```python
from build123d import *

# Parameters (mm, degrees)
SKETCH1_W           = 31
SKETCH1_H           = 26
BOSS_EXTRUDE1_DEPTH = 1.2
SKETCH3_W           = 1.2
SKETCH3_H           = 26
BOSS_EXTRUDE2_DEPTH = 33
SKETCH4_R           = 3.5
CUT_EXTRUDE1_DEPTH  = 1.2
SKETCH2_R           = 5
SKETCH2_R_2         = 2
CUT_EXTRUDE2_DEPTH  = 1.2
FILLET1_R           = 1
FILLET2_R           = 3


with BuildPart() as part:
    # Sketch1 → Boss-Extrude1 (new body)
    with BuildSketch(Plane(origin=(0, 0, 0), x_dir=(1, 0, 0), z_dir=(0, 1, 0))):
        Rectangle(SKETCH1_W, SKETCH1_H)
    extrude(amount=BOSS_EXTRUDE1_DEPTH)

    # Sketch3 → Boss-Extrude2 (add)
    with BuildSketch(Plane.XZ):
        with Locations((14.9, 0)):
            Rectangle(SKETCH3_W, SKETCH3_H)
    extrude(amount=BOSS_EXTRUDE2_DEPTH)

    # Sketch4 → Cut-Extrude1 (cut)
    with BuildSketch(Plane(origin=(15.5, 0, 0), x_dir=(0, 0, -1), z_dir=(1, 0, 0))):
        with BuildLine():
            Line((13, -33), (13, -20))
            ThreePointArc((13, -20), (9.192388155, -29.192388155), (0, -33))
            Line((0, -33), (13, -33))
        make_face()
        with BuildLine():
            Line((-13, -33), (0, -33))
            ThreePointArc((0, -33), (-9.192388155, -29.192388155), (-13, -20))
            Line((-13, -20), (-13, -33))
        make_face()
        with Locations((0, -20)):
            Circle(SKETCH4_R)
    extrude(amount=-CUT_EXTRUDE1_DEPTH, mode=Mode.SUBTRACT)

    # Sketch2 → Cut-Extrude2 (cut)
    with BuildSketch(Plane(origin=(0, 1.2, 0), x_dir=(1, 0, 0), z_dir=(0, 1, 0))):
        with Locations(Location((0, 0, 0), (0, 0, 270))):
            Circle(SKETCH2_R)
        with Locations(Location((-7.5, 8, 0), (0, 0, 270))):
            Circle(SKETCH2_R_2)
        with Locations(Location((6.5, 8, 0), (0, 0, 270))):
            Circle(SKETCH2_R_2)
        with Locations(Location((6.5, -8, 0), (0, 0, 90))):
            Circle(SKETCH2_R_2)
        with Locations(Location((-7.5, -8, 0), (0, 0, 90))):
            Circle(SKETCH2_R_2)
    extrude(amount=-CUT_EXTRUDE2_DEPTH, mode=Mode.SUBTRACT)

    # Fillet1
    fillet1_edges = [part.edges().sort_by_distance(p)[0] for p in [
        (15.5, 1.2, 0),
        (14.3, 0, 0),
    ]]
    fillet(fillet1_edges, radius=FILLET1_R)

    # Fillet2
    fillet2_edges = [part.edges().sort_by_distance(p)[0] for p in [
        (-15.5, 0.6, -13),
        (-15.5, 0.6, 13),
    ]]
    fillet(fillet2_edges, radius=FILLET2_R)


solid = part.part
```
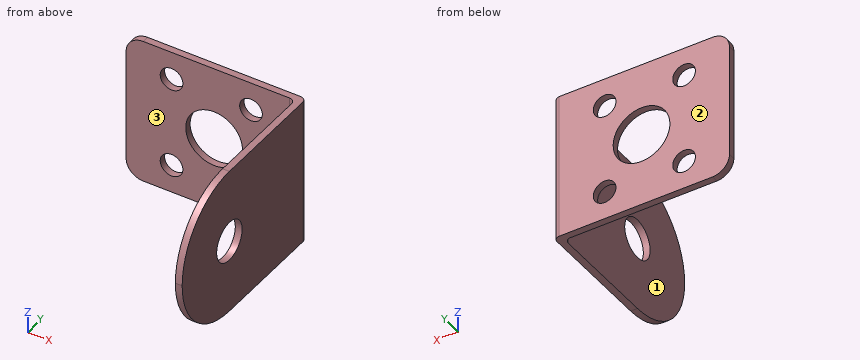
Can you work these out from the model? Positions are in its coordinate system, mm. Face numbers are marked on the shaded views. Coordinates: 2 decimals unless noted, no trailing zeros. Order: outer loops, then holes, each group sorted by start corner. A loop starts at its lowest first (then second) coordinate and runs counter-clockwise, first axis right, second up. Notation, with made-up numbers: (-29, -32.5) -> (-6, -32.5) arc R35 ccw to (-6, 2.5) -> close; hole circle Ø7 at (-39.75, 86). An arc over 180 degrees is marked (long way). Write each question's results on one line, items separated by ' | '.
Item 1: I want a section at A-A, the plane y = -18.5. Write out the boundary of the cut face in (x, z).
Results are:
outline: (14.3, -13) -> (15.5, -13) -> (15.5, -3.16) -> (14.3, -3.16) -> close; (14.3, 3.16) -> (15.5, 3.16) -> (15.5, 13) -> (14.3, 13) -> close
Item 2: If I drill on line 1 along X through (y, z) = (0.35, 8); line 2 along X through (y, z) = (0.8, 8); line 3 along Y through (x, z) = (-2.5, 8.25), over which ranges is the centre line in solid material (lowest first)?
Results are:
line 1: -15.5 to -9.5, -5.5 to 4.5, 8.5 to 15.49 | line 2: -15.5 to -9.5, -5.5 to 4.5, 8.5 to 15.3 | line 3: 0 to 1.2
Item 3: I want a section at D-D, the plane x = -10. Write out the boundary of the cut face in (y, z), then the cut area to 3 significant figures.
Results are:
outline: (0, -13) -> (1.2, -13) -> (1.2, 13) -> (0, 13) -> close | area: 31.2 mm²
Item 4: I'm going to push flat-ended pins straight in: pin 1 Ø12 at (y, z) = (-21.5, -5.5) entering from -X; pin 2 Ø3 at (x, z) = (-7.5, 8) entering from +Y; pin 3 Ø8 at (x, z) = (-1, 2) entering from -Y. Where does each tip first touch, or does it pass through?
Results are:
pin 1: x = 14.3 | pin 2: through | pin 3: y = 0
Item 5: I want a section at C-C, the plane x = 6.5. Write out the boundary of the cut face in (y, z).
Results are:
outline: (0, -13) -> (1.2, -13) -> (1.2, -10) -> (0, -10) -> close; (0, -6) -> (1.2, -6) -> (1.2, 6) -> (0, 6) -> close; (0, 10) -> (1.2, 10) -> (1.2, 13) -> (0, 13) -> close
Item 6: If we mould it in two halves opening along Y, with no side actions, what happens to the marked faces 1, 2 and 3? For each: +Y half, -Y half, draft (parallel to the pull), parting line (faces both ways), or undercut.
Results are:
face 1: draft | face 2: +Y half | face 3: -Y half
Item 7: I want a section at B-B, the plane z = 7. Write out the boundary of the cut face in (x, y), then the cut area to 3 significant figures.
Results are:
outline: (-15.5, 0) -> (-9.23, 0) -> (-9.23, 1.2) -> (-15.5, 1.2) -> close; (-5.77, 0) -> (4.77, 0) -> (4.77, 1.2) -> (-5.77, 1.2) -> close; (8.23, 0) -> (13.3, 0) arc R1 cw to (14.3, -1) -> (14.3, -30.95) -> (15.5, -30.95) -> (15.5, 0.2) arc R1 ccw to (14.5, 1.2) -> (8.23, 1.2) -> close | area: 66.0 mm²
